Job drawing, mm, ordinate dimensions from the low corner. One solid piece. A direction names the side the tool comes from. Give positions to 0.01 mm unless a question says otherwise; leave off trailing zeros. Write each loop counter-clockwise with the first axis right and the second up, starting at its lowest first coordinate (ties: lowest second). Pieces come first, ordered by that corner, then holes. Notation, with made-up numbers: (-5.5, -33) -> (2.5, -33) arc R19 cw to (2.5, 2) -> close; hole circle Ø10 at (9.25, 53). An arc over 180 degrees is marked (long way). Put each result on its own line as item: value. Start each with the question number.
Item 1: Slice it at A-A, the plane x = 8.5. List the corners of the cut face in (y, z), plus the area to 3 significant figures.
Item 2: Slice it at C-C, the plane z = 13.5. List the corners of the cut face in (x, y).
Item 3: Flat gauge pins, fed straight in: pin 1 Ø5 at (x, y) = (7, 8) entering from +Z; pin 2 Ø0.9 at (x, z) = (8, 11) entering from -Y; pin 3 Ø4 at (x, z) = (5.5, 3.5) entering from -Y; pin 4 Ø3 at (y, z) = (2, 12) entering from +X (3 decimals). Where does each tip first touch, or does it go through?
Item 4: Tool access for the marked faces 1, 2 and 3: list every direction of +Z, -Z, +X, -X, +Y, -Y with a clear straight run to the whole face (end or side of a thin tool).
Item 5: Slice it at D-D, the plane y = 10.75. List the corners of the cut face in (x, z), plus the area to 3 significant figures.
Item 6: Slice it at B-B, the plane y = 7.75. List the corners of the cut face in (x, z), plus the area to 3 significant figures.
Item 7: Drill centre lines: line 1 along X through (y, z) = (8.5, 5.75); line 2 along Z through (x, y) = (4.1, 8.5); line 3 along X through (y, z) = (8.5, 3.75). Where is each one in solid material? Low to high.
Item 8: Two-plate mould, pull along Z, no slides. Class the marked faces 4, 5, 6 and 7: pulls with the +Z half, pulls with the -Z half, needs draft (parallel to the pull), parting line crosses it, or undercut.
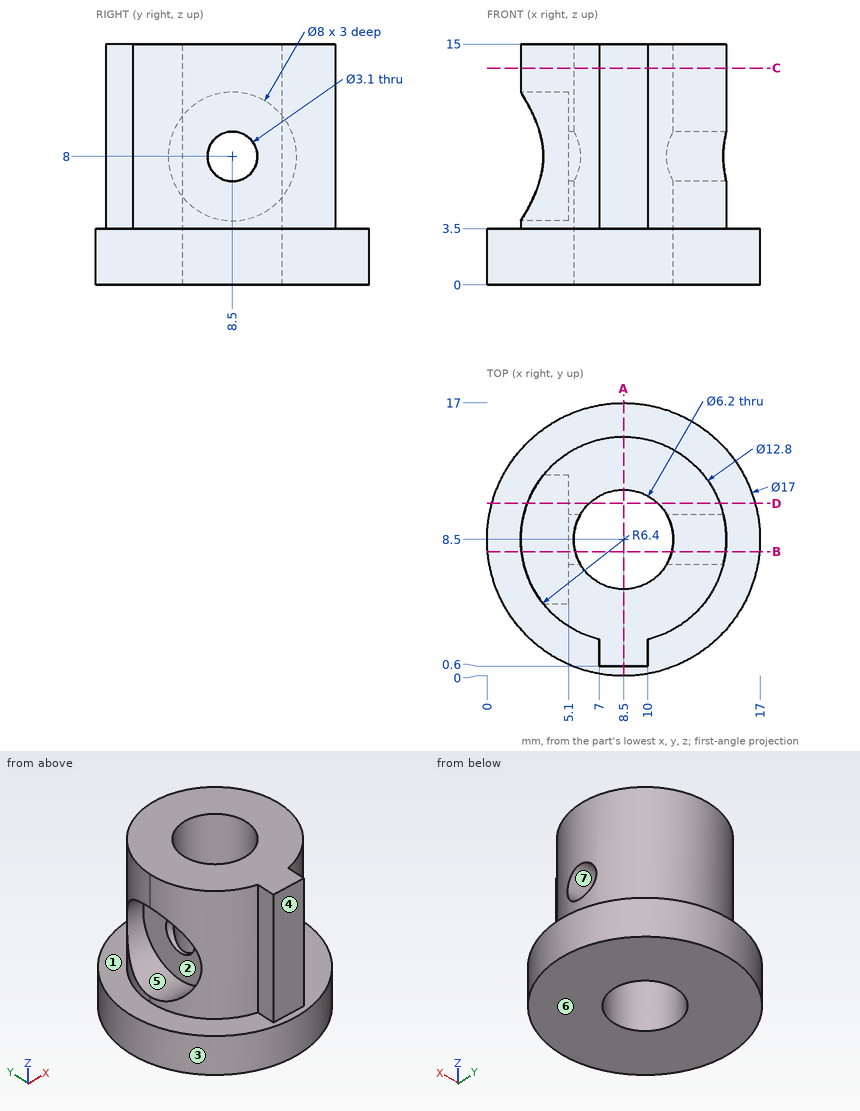
Values follow:
1. outline: (0, 0) -> (5.4, 0) -> (5.4, 15) -> (0.6, 15) -> (0.6, 3.5) -> (0, 3.5) -> close; (11.6, 0) -> (17, 0) -> (17, 3.5) -> (14.9, 3.5) -> (14.9, 15) -> (11.6, 15) -> close
1. area: 131 mm2
2. outline: (7, 0.6) -> (10, 0.6) -> (10, 2.28) arc R6.4 ccw (long way) to (7, 2.28) -> close; hole circle Ø6.2 at (8.5, 8.5)
3. pin 1: z = 15
3. pin 2: y = 0.6
3. pin 3: y = 0.06
3. pin 4: x = 12.495
4. face 1: +Z
4. face 2: -X
4. face 3: +Z, -Z
5. outline: (0.3, 0) -> (6.37, 0) -> (6.37, 15) -> (2.51, 15) -> (2.51, 11.31) -> (5.1, 11.31) -> (5.1, 4.69) -> (2.51, 4.69) -> (2.51, 3.5) -> (0.3, 3.5) -> close; (10.63, 0) -> (16.7, 0) -> (16.7, 3.5) -> (14.49, 3.5) -> (14.49, 15) -> (10.63, 15) -> close
5. area: 114 mm2
6. outline: (0.03, 0) -> (5.49, 0) -> (5.49, 6.64) -> (5.1, 6.64) -> (5.1, 4.07) -> (2.14, 4.07) -> (2.14, 3.5) -> (0.03, 3.5) -> close; (2.14, 11.93) -> (5.1, 11.93) -> (5.1, 9.36) -> (5.49, 9.36) -> (5.49, 15) -> (2.14, 15) -> close; (11.51, 0) -> (16.97, 0) -> (16.97, 3.5) -> (14.86, 3.5) -> (14.86, 6.64) -> (11.51, 6.64) -> close; (11.51, 9.36) -> (14.86, 9.36) -> (14.86, 15) -> (11.51, 15) -> close
6. area: 81.8 mm2
7. line 1: 5.1 to 5.4, 11.6 to 14.9
7. line 2: 0 to 4, 12 to 15
7. line 3: 2.1 to 5.4, 11.6 to 14.9
8. face 4: needs draft
8. face 5: undercut
8. face 6: pulls with the -Z half
8. face 7: undercut
